Verification items for the finished model (mm, model axes). Give positions to 0.01 mm unless a question says otherwise; leave off trailing zeros. Loops run counter-clockwise (first coordinate to the right, second up) from the corner with the lowest first, then second, coordinate; pieces in that order, holes last. Notation, with made-up numbers: (20.25, 71.25) - (64.25, 71.25) arc R17 ccw to (64.25, 104.25) - close; hole circle Ø5 at (-22.75, 84.25). An arc over 180 degrees is marked (long way). One line per question, with ' | ' between items. Start each with the question number.
1. Section check A-A, the plane y = 1.3. Enter the section's corners in (x, z).
2. Mould release check, pull along X, two halves, no side actions. Record for faces 1 (the face through (0.631, 1.972, -2.003)), 2 (the face through (2.083, 3.915, -3.587)), 3 (the face through (-3.448, 1.972, -2.028)): +X half, -X half, draft (parallel to the pull), parting line (faces both ways), or undercut.
3. Thickness scan on line 1 along X through (y, z) = (3.5, -1.25); line 2 along X through (y, z) = (0.9, 1.75); line 3 along Z through (x, y) = (0.5, 3.8). Record the ranges inside material, lowest first. Write a range as from..to.
4. Depth check by flat-ended pin: pin 1 Ø2 at (x, z) = (-0.5, 1.5) entering from +Y; pin 2 Ø1.5 at (y, z) = (1.5, 1) entering from -X. Enter the tip coordinate at first touch or a pass-through.
from build123d import *

# Parameters (mm, degrees)
BOSS_EXTRUDE1_DEPTH = 4
M5_TAPPED_HOLE1_D   = 4.2


with BuildPart() as part:
    # Sketch1 → Boss-Extrude1 (new body)
    with BuildSketch(Plane(origin=(0, 0, 0), x_dir=(1, 0, 0), z_dir=(0, 1, 0))):
        Polygon((-2.309401077, -4), (2.309401077, -4), (4.618802154, 0), (2.309401077, 4), (-2.309401077, 4), (-4.618802154, 0), align=None)
    extrude(amount=BOSS_EXTRUDE1_DEPTH)

    # Sketch2 → Cut-Revolve1 (revolve, cut)
    with BuildSketch(Plane(origin=(0, 0, 0), x_dir=(0, 0, -1), z_dir=(1, 0, 0))):
        Polygon((5.752238375, 1.011655298), (4, 0), (5.752238375, 0), align=None)
        Polygon((4, 4), (6.116124346, 4), (6.116124346, 2.778255039), align=None)
    revolve(axis=Axis((0, 0, 0), (0, 1, 0)), mode=Mode.SUBTRACT)

    # M5 Tapped Hole1 (through all)
    with Locations(Plane.ZX.offset(4)):
        with Locations((0, 0)):
            Hole(M5_TAPPED_HOLE1_D / 2)


solid = part.part
Results list:
1) outline: (-4.62, 0) - (-2.31, -4) - (2.31, -4) - (4.62, 0) - (2.31, 4) - (-2.31, 4) - close; hole circle Ø4.2 at (0, 0)
2) face 1: undercut | face 2: +X half | face 3: -X half
3) line 1: -3.9..-1.69, 1.69..3.9 | line 2: -3.61..-1.16, 1.16..3.61 | line 3: -4..-2.04, 2.04..4
4) pin 1: y = 4 | pin 2: x = -4.47
